```python
from build123d import *

# Parameters (mm, degrees)
SKETCH1_W            = 174
SKETCH1_H            = 65
BOSS_EXTRUDE1_DEPTH  = 3
SKETCH2_R            = 4
SKETCH2_R_2          = 5.75
SKETCH2_W            = 28
SKETCH2_H            = 15
SKETCH2_W_2          = 11
CUT_EXTRUDE1_DEPTH   = 3
SKETCH3_R            = 1.25
BOSS_EXTRUDE2_DEPTH  = 3.5
LPATTERN1_COUNT      = 2
LPATTERN1_PITCH      = 171
LPATTERN1_COUNT_DIR2 = 2
LPATTERN1_PITCH_DIR2 = 62


with BuildPart() as part:
    # Sketch1 → Boss-Extrude1 (new body)
    with BuildSketch(Plane(origin=(0, 0, 0), x_dir=(1, 0, 0), z_dir=(0, 1, 0))):
        with Locations((22.975352113, 1.809859155)):
            Rectangle(SKETCH1_W, SKETCH1_H)
    extrude(amount=BOSS_EXTRUDE1_DEPTH)

    # Sketch2 → Cut-Extrude1 (cut)
    with BuildSketch(Plane(origin=(0, 3, 0), x_dir=(1, 0, 0), z_dir=(0, 1, 0))):
        with Locations(Location((37.975352113, 1.809859155, 0), (0, 0, 270))):
            Circle(SKETCH2_R)
        with Locations(Location((-8.024647887, 1.809859155, 0), (0, 0, 270))):
            Circle(SKETCH2_R_2)
        with Locations((16.475352113, 1.809859155)):
            Rectangle(SKETCH2_W, SKETCH2_H)
        with Locations((-24.024647887, 1.809859155)):
            Rectangle(SKETCH2_W_2, SKETCH2_H)
    extrude(amount=-CUT_EXTRUDE1_DEPTH, mode=Mode.SUBTRACT)

    # Sketch3 → Boss-Extrude2 (add)
    with BuildSketch(Plane.XZ):
        with Locations(Location((-62.434647887, -32.719859155, 0), (0, 0, 90))):
            Circle(SKETCH3_R)
    boss_extrude2 = extrude(amount=BOSS_EXTRUDE2_DEPTH)

    # LPattern1: Boss-Extrude2 2 × 2
    with Locations(*[(i * LPATTERN1_PITCH, 0, j * LPATTERN1_PITCH_DIR2) for i in range(LPATTERN1_COUNT) for j in range(LPATTERN1_COUNT_DIR2) if (i, j) != (0, 0)]):
        add(boss_extrude2)


solid = part.part
```
The listing builds one solid part. Answer for the finished solid, in the listing's coordinates (mm). A direction names the side the tool comes from. Round coordinates to 2 decimals unless told otherwise and drop trailing zeros. Order: outer loops, then holes, each group sorted by start corner. A loop starts at its lowest first (then second) coordinate and runs counter-clockwise, first axis right, second up. Notation, with made-up numbers: (-22.5, 74) -> (-8.5, 74) arc R22 cw to (-8.5, 93) -> close; hole circle Ø9 at (83, 48.5). An arc over 180 degrees is marked (long way). Answer as CSV lines item,"result". Start each with the question number.
(1) The part is cut by section C-C (z = 14.5). Determine the outline of the cut face in (x, y), then the cut area to 3 significant figures.
(2) The part is cut by section A-A (x = 14). Determine the outline of the cut face in (y, z), then the cut area to 3 significant figures.
(3) For a pull along Z with two mould halves and no side action, classify faces 1 (the face through (16, 2, 5.69)), 2 (the face through (22, 1, -34.31)), 3 (the face through (-64.025, 1, -1)) as +Z half, -Z half, draft (parallel to the pull), parting line (faces both ways), or undercut.
(4) The part is cut by section D-D (x = -40.5). Determine the outline of the cut face in (y, z), then the cut area to 3 significant figures.
(5) The part is cut by section B-B (y = 1.5). Determine the outline of the cut face in (x, z).
(6) Find the intervals of material crossed by probe 1 along Y at (x, z) = (-33, 23.5); probe 2 along Z at (x, y) = (4.5, 1.25), in increasing order. Write a range as from..to.
(7) A flat-ended cylindrical pin translates along its axis: pin 1 Ø3 at (x, z) = (4, -9.5) entering from -Y. Find the tip coordinate at first contact, or state that the pin passes through.
(8) A tool of negligible diameter and unlimited length cuts with its end or side. For faces 4 (the face through (30.475, 2, -2)), 5 (the face through (22, 1, 30.69)), from which of +Z, -Z, +X, -X, +Y, -Y can it reach the whole face along a straight path? Write none if from no direction.
Evaluation:
1,outline,"(-64.02, 0) -> (109.98, 0) -> (109.98, 3) -> (-64.02, 3) -> close"
1,area,"522 mm²"
2,outline,"(0, -34.31) -> (3, -34.31) -> (3, -9.31) -> (0, -9.31) -> close; (0, 5.69) -> (3, 5.69) -> (3, 30.69) -> (0, 30.69) -> close"
2,area,"150 mm²"
3,face 1,"undercut"
3,face 2,"-Z half"
3,face 3,"draft"
4,outline,"(0, -34.31) -> (3, -34.31) -> (3, 30.69) -> (0, 30.69) -> close"
4,area,"195 mm²"
5,outline,"(-64.02, -34.31) -> (109.98, -34.31) -> (109.98, 30.69) -> (-64.02, 30.69) -> close; hole (-29.52, -9.31) -> (-18.52, -9.31) -> (-18.52, 5.69) -> (-29.52, 5.69) -> close; hole circle Ø11.5 at (-8.02, -1.81); hole (2.48, -9.31) -> (30.48, -9.31) -> (30.48, 5.69) -> (2.48, 5.69) -> close; hole circle Ø8 at (37.98, -1.81)"
6,probe 1,"0..3"
6,probe 2,"-34.31..-9.31, 5.69..30.69"
7,pin 1,"y = 0"
8,face 4,"+Y, -Y"
8,face 5,"+Z, +X, -X, +Y, -Y"
